The model under review builds one solid part; all positions refer to its coordinate system, in mm. Face numbers are marked on the shaded views. A direction names the side the tool comes from. Give positions to 0.01 mm unless a question says otherwise; leave off trailing zeros. Loops run counter-clockwise (first coordinate to the right, second up) from the corner with the lowest first, then second, coordinate; pieces in that order, holes last. Notation, with made-up numbers: M -39.75,51.25 L -3.75,51.25 A13 cw -3.75,61.25 Z; hole C 70.5,-28.75 d2. An arc over 180 degrees is marked long. Write item = value, one per line. Start each with the question number.
1. For pin 1 (3.5 mm diameter, centred on x = 0, y = -9.5, fed in from -Z); pin 2 (2 mm diameter, centred on x = -2.5, z = 2, fed in from -Y); pin 3 (4 mm diameter, centred on y = 5, z = 8, fed in from +X), all flat-tipped, find the tip position at first contact; note any pin that passes through.
2. We need section A-A on x = 0. Give the boundary of the cut face in (y, z), then the cut area to 3 significant figures.
3. For the marked faces 4 and 5, list the 3-axis set-ups (+Z, -Z, +X, -X, +Y, -Y) from which the entire face can be reached by the end or side of a thin tool; tool diameter is ignored.
4. Draft analysis for pull direction X (two halves, no side actions). For the marked faces 1, 2 and 3, state which applies: pulls with the +X half, pulls with the -X half, needs draft (parallel to the pull), parting line crosses it, or undercut.
5. We need section D-D on y = -10.5. Give the boundary of the cut face in (x, z).
6. Wall thickness on line 1 along Y through (x, z) = (0, 5.6); line 2 along Y through (x, z) = (0, 4); line 3 along Z through (x, y) = (-9.25, -5): over which ranges is each line inside the solid? List them lowest first. Write a range as from..to.
7. We need section C-C on x = -9.5. Give the boundary of the cut face in (y, z).
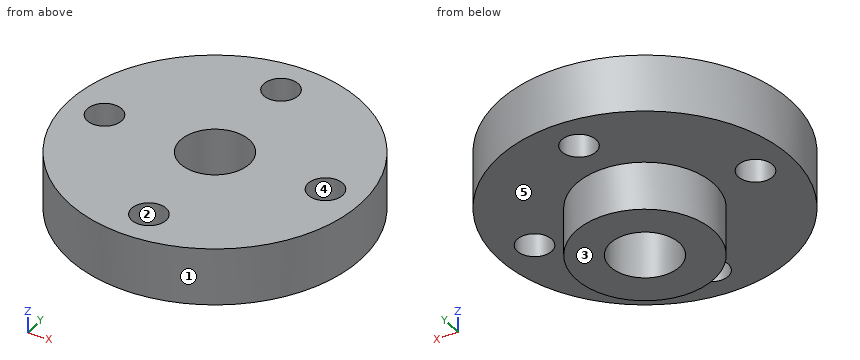
from build123d import *

# Parameters (mm, degrees)
SKETCH1_R           = 6
SKETCH1_R_2         = 3
BOSS_EXTRUDE1_DEPTH = 4.2
SKETCH2_R           = 12.7
SKETCH2_R_2         = 3
BOSS_EXTRUDE2_DEPTH = 5
SKETCH3_R           = 1.5
CUT_EXTRUDE1_DEPTH  = 5


with BuildPart() as part:
    # Sketch1 → Boss-Extrude1 (new body)
    with BuildSketch(Plane.XY):
        Circle(SKETCH1_R)
        Circle(SKETCH1_R_2, mode=Mode.SUBTRACT)
    extrude(amount=BOSS_EXTRUDE1_DEPTH)

    # Sketch2 → Boss-Extrude2 (add)
    with BuildSketch(Plane.XY.offset(4.2)):
        Circle(SKETCH2_R)
        Circle(SKETCH2_R_2, mode=Mode.SUBTRACT)
    extrude(amount=BOSS_EXTRUDE2_DEPTH)

    # Sketch3 → Cut-Extrude1 (cut)
    with BuildSketch(Plane.XY.offset(9.2)):
        with Locations((0, 9.49515399)):
            Circle(SKETCH3_R)
        with Locations((0, -9.5)):
            Circle(SKETCH3_R)
        with Locations((9.5, 0)):
            Circle(SKETCH3_R)
        with Locations((-9.5, 0)):
            Circle(SKETCH3_R)
    extrude(amount=-CUT_EXTRUDE1_DEPTH, mode=Mode.SUBTRACT)


solid = part.part
Final values:
q1.pin_1 = 4.2
q1.pin_2 = -5.81
q1.pin_3 = 12.34
q2.outline = M -12.7,4.2 L -11,4.2 L -11,9.2 L -12.7,9.2 Z; M -8,4.2 L -6,4.2 L -6,0 L -3,0 L -3,9.2 L -8,9.2 Z; M 3,0 L 6,0 L 6,4.2 L 8,4.2 L 8,9.2 L 3,9.2 Z; M 11,4.2 L 12.7,4.2 L 12.7,9.2 L 11,9.2 Z
q2.area = 92.2 mm²
q3.face_4 = +Z, -Z
q3.face_5 = -Z
q4.face_1 = parting line crosses it
q4.face_2 = undercut
q4.face_3 = needs draft
q5.outline = M -7.14,4.2 L -1.12,4.2 L -1.12,9.2 L -7.14,9.2 Z; M 1.12,4.2 L 7.14,4.2 L 7.14,9.2 L 1.12,9.2 Z
q6.line_1 = -12.7..-11, -8..-3, 3..8, 11..12.7
q6.line_2 = -6..-3, 3..6
q6.line_3 = 4.2..9.2
q7.outline = M -8.43,4.2 L -1.5,4.2 L -1.5,9.2 L -8.43,9.2 Z; M 1.5,4.2 L 8.43,4.2 L 8.43,9.2 L 1.5,9.2 Z
